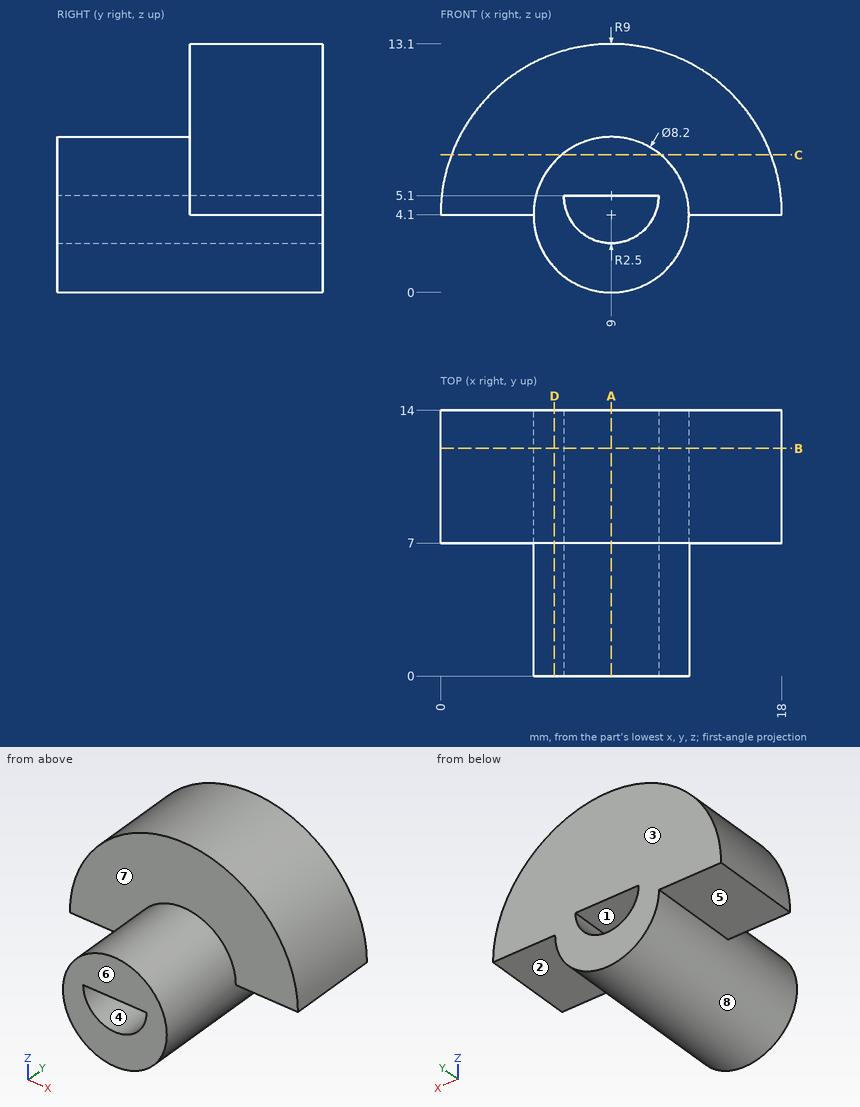
Study the drawing (mm; zero at the part's minimum x, y, z) and answer. A direction names the side the tool comes from. Coordinates: 2 decimals unless noted, no trailing zeros. Loops run counter-clockwise (first coordinate to the right, second up) from the corner with the lowest first, then second, coordinate; pieces in that order, holes last. Notation, with made-up numbers: M 24,72 L 36,72 A27 cw 36,91 Z; hole C 58,55 d4. An arc over 180 degrees is marked long. Answer in a Markdown table with one row per item. Add a question column.
1. The mould has two halves that part along Z. Classify the marked faces 1, 2, 3 and 4: pulls with the +Z half, pulls with the -Z half, needs draft (parallel to the pull), parting line crosses it, or undercut.
2. Find section A-A, the plane x = 9. Write down the section's boundary in (y, z), then the cut area to 3 significant figures.
3. Find section B-B, the plane y = 12. Write down the section's boundary in (x, z).
4. Find section C-C, the plane z = 7.25. Write down the section's boundary in (x, y).
5. Flat-ended cylindrical pins translate along their axes: P1, Ø2.5, axis at x = 3, y = 12, coming from the -Z side; P2, Ø1.5, axis at y = 9, z = 2, coming from the +X side; P3, Ø4, axis at y = 7.5, z = 6.5, coming from the -X side. Find the tip coordinate at first contact, or state that the pin passes through.
6. Find section D-D, the plane x = 6. Write down the section's boundary in (y, z).
7. A tool of negligible diameter and unlimited length cuts with its end or side. For the marked faces 5, 6, 7 and 8, from which of +Z, -Z, +X, -X, +Y, -Y can it reach the whole face along a straight path? Write none if from no direction.
8. Consider L1, parallel to X at y = 9.25, z = 4 (3 decimals); L2, parallel to Y at x = 6.5, z = 8.25; L3, parallel to Z at x = 10.5, y = 4. Determine where each line is inside the solid, lowest interval first.
Reported:
| question | item | result |
|---|---|---|
| 1 | face 1 | undercut |
| 1 | face 2 | pulls with the -Z half |
| 1 | face 3 | needs draft |
| 1 | face 4 | undercut |
| 2 | outline | M 0,0 L 14,0 L 14,2.6 L 0,2.6 Z; M 0,5.1 L 14,5.1 L 14,13.1 L 7,13.1 L 7,8.2 L 0,8.2 Z |
| 2 | area | 114 mm^2 |
| 3 | outline | M 0,4.1 L 4.9,4.1 A4.1 ccw 13.1,4.1 L 18,4.1 A9 ccw Z; hole M 6.5,5.1 A2.5 ccw 11.5,5.1 Z |
| 4 | outline | M 0.57,7 L 6.38,7 L 6.38,0 L 11.62,0 L 11.62,7 L 17.43,7 L 17.43,14 L 0.57,14 Z |
| 5 | P1 | stops at z = 4.1 |
| 5 | P2 | stops at x = 12.87 |
| 5 | P3 | stops at x = 0.01 |
| 6 | outline | M 0,1.31 L 14,1.31 L 14,12.59 L 7,12.59 L 7,6.89 L 0,6.89 Z |
| 7 | face 5 | -Z, -X, +Y, -Y |
| 7 | face 6 | +Z, -Z, +X, -X, -Y |
| 7 | face 7 | +Z, -Y |
| 7 | face 8 | -Y |
| 8 | L1 | x = 4.901 to 6.755, 11.245 to 13.099 |
| 8 | L2 | y = 7 to 14 |
| 8 | L3 | z = 0.28 to 3.1, 5.1 to 7.92 |
